Model file for the job. Use its own axes, mm. A direction names the side the tool comes from. Coordinates: 2 decimals unless noted, no trailing zeros. Write each loop counter-clockwise with the first axis right and the second up, starting at its lowest first coordinate (ties: lowest second). Pieces come first, ordered by that corner, then holes. Notation, with made-up numbers: (-23.75, 20.5) - (30.25, 20.5) arc R16 cw to (30.25, 24.5) - close; hole circle Ø5 at (51.5, -20.75). An arc over 180 degrees is marked (long way). Put each result on its own line as item: value. Start each with the question number.
1. Drop flat-ended pins along their axis: P1, Ø5, axis at x = 3.5, z = -1, coming from the -Y side; P2, Ø2, axis at x = 4, z = 0.5, coming from the -Y side; P3, Ø4, axis at x = 1, z = 2, coming from the -Y side; P4, Ø1.1, axis at y = -5, z = 0, coming from the -X side. Give the stop position or say it passes through.
2. Saw through at A-A, the plane x = -2. Write the cut outline in (y, z).
3. Pull direction X, two halves, no side cores. Call faces 5 (the face through (-5.64, -6.99, 2.15)), 6 (the face through (-4.75, -4, -1)), 7 (the face through (0, 7, -3)): released by +X, released by -X, zero draft, split by the parting line, or undercut.
4. Saw through at C-C, the plane z = 1.25. Write the cut outline in (x, y), plus the area to 3 significant figures.
5. Drill centre lines: L1, parallel to Z at x = -3.75, y = 1.5; L2, parallel to X at y = 3, z = 4; L3, parallel to X at y = 2.75, z = 2.5. Where is each one in solid material? Low to high. Write a range as from..to.
6. Saw through at B-B, the plane y = 6.25. Write the cut outline in (x, z).
7. Saw through at D-D, the plane y = -3.5. Write the cut outline in (x, z).
8. Which spindle directions (+Z, -Z, +X, -X, +Y, -Y) get a long thin tool onto all of the face, cutting with end or side? Do faces 1 (the face through (4.5, 8, 0)), 2 (the face through (4.75, -4, -1)), 3 (the face through (0, 5, -5)), 4 (the face through (4, 5, 4)). Say none if no direction does.
```python
from build123d import *

# Parameters (mm, degrees)
SKETCH1_W               = 13
SKETCH1_H               = 10
SKETCH1_W_2             = 9
SKETCH1_H_2             = 6
BOSS_EXTRUDE1_DEPTH     = 15
BOSS_EXTRUDE2_DEPTH     = 2
SKETCH3_R               = 0.95
CUT_EXTRUDE1_DEPTH      = 14
SKETCH5_W               = 0.25
SKETCH5_H               = 10
CUT_EXTRUDE3_DEPTH      = 6
CUT_EXTRUDE3_DEPTH_BACK = 6
SKETCH6_W               = 8
SKETCH6_H               = 0.8
CUT_EXTRUDE4_DEPTH      = 10


with BuildPart() as part:
    # Sketch1 → Boss-Extrude1 (new body)
    with BuildSketch(Plane(origin=(0, 0, 0), x_dir=(1, 0, 0), z_dir=(0, 1, 0))):
        Rectangle(SKETCH1_W, SKETCH1_H)
        Rectangle(SKETCH1_W_2, SKETCH1_H_2, mode=Mode.SUBTRACT)
    extrude(amount=BOSS_EXTRUDE1_DEPTH)

    # Sketch2 → Boss-Extrude2 (add)
    with BuildSketch(Plane(origin=(6.5, 0, 0), x_dir=(0, 0, -1), z_dir=(1, 0, 0))):
        with BuildLine():
            ThreePointArc((-5, 0), (-2.071067812, -7.071067812), (5, -10))
            Line((5, -10), (5, 0))
            Line((5, 0), (-5, 0))
        make_face()
    boss_extrude2 = extrude(amount=-BOSS_EXTRUDE2_DEPTH)

    # Mirror1: Boss-Extrude2 across plane
    add(boss_extrude2.mirror(Plane(origin=(0, 0, 0), x_dir=(0, 0, 1), z_dir=(1, 0, 0))))

    # Sketch3 → Cut-Extrude1 (cut, through all)
    with BuildSketch(Plane(origin=(6.5, 0, 0), x_dir=(0, 0, -1), z_dir=(1, 0, 0))):
        with Locations((0, -5)):
            Circle(SKETCH3_R)
    extrude(amount=-CUT_EXTRUDE1_DEPTH, mode=Mode.SUBTRACT)

    # Sketch5 → Cut-Extrude3 (cut, two sides)
    with BuildSketch(Plane.XY) as cut_extrude3_sk:
        with Locations((-4.625, -5)):
            Rectangle(SKETCH5_W, SKETCH5_H)
        with Locations((4.625, -5)):
            Rectangle(SKETCH5_W, SKETCH5_H)
    extrude(amount=CUT_EXTRUDE3_DEPTH, mode=Mode.SUBTRACT)
    extrude(cut_extrude3_sk.sketch, amount=-CUT_EXTRUDE3_DEPTH_BACK, mode=Mode.SUBTRACT)

    # Sketch6 → Cut-Extrude4 (cut)
    with BuildSketch(Plane.XZ):
        with Locations((0, 4)):
            Rectangle(SKETCH6_W, SKETCH6_H)
    cut_extrude4 = extrude(amount=-CUT_EXTRUDE4_DEPTH, mode=Mode.SUBTRACT)

    # Mirror2: Cut-Extrude4 across plane
    add(cut_extrude4.mirror(Plane.XY), mode=Mode.SUBTRACT)


solid = part.part
```
Final values:
1. P1: stops at y = -9.83
1. P2: stops at y = -8.75
1. P3: stops at y = 0
1. P4: passes through
2. outline: (0, -5) - (15, -5) - (15, -3) - (0, -3) - (0, -3.6) - (10, -3.6) - (10, -4.4) - (0, -4.4) - close; (0, 3) - (15, 3) - (15, 5) - (0, 5) - (0, 4.4) - (10, 4.4) - (10, 3.6) - (0, 3.6) - close
3. face 5: zero draft
3. face 6: undercut
3. face 7: undercut
4. outline: (-6.5, -7.81) - (-4.75, -7.81) - (-4.75, 0) - (-4.5, 0) - (-4.5, 15) - (-6.5, 15) - close; (4.5, 0) - (4.75, 0) - (4.75, -7.81) - (6.5, -7.81) - (6.5, 15) - (4.5, 15) - close
4. area: 87.3 mm²
5. L1: z = -5..-4.4, -3.6..-3, 3..3.6, 4.4..5
5. L2: x = -6.5..-4, 4..6.5
5. L3: x = -6.5..-4.5, 4.5..6.5
6. outline: (-6.5, -5) - (6.5, -5) - (6.5, 5) - (-6.5, 5) - close; hole (-4.5, -3) - (4.5, -3) - (4.5, 3) - (-4.5, 3) - close; hole (-4, -4.4) - (4, -4.4) - (4, -3.6) - (-4, -3.6) - close; hole (-4, 3.6) - (4, 3.6) - (4, 4.4) - (-4, 4.4) - close
7. outline: (-6.5, -5) - (-4.75, -5) - (-4.75, 4.37) - (-6.5, 4.37) - close; (4.75, -5) - (6.5, -5) - (6.5, 4.37) - (4.75, 4.37) - close
8. face 1: +Y, -Y
8. face 2: +Z, -Z, -Y
8. face 3: -Z, +X, -X, +Y, -Y
8. face 4: -Y
